Verification items for the finished model (mm, model axes). A direction names the side the tool comes from. Coordinates: 2 decimals unless noted, no trailing zeros. Order: outer loops, then holes, each group sorted by start corner. A loop starts at its lowest first (then second) coordinate and runs counter-clockwise, first axis right, second up. Notation, with made-up numbers: M 37,67 L 76,67 A31 ccw 76,98 Z; hole C 6,4.25 d7. An arc over 180 degrees is marked long. Write item = value, one per line.
```python
from build123d import *

# Parameters (mm, degrees)
F0_R          = 1.5
F1_DEPTH      = 2
F2_W          = 18
F2_H          = 8
F2_W_2        = 14
F2_H_2        = 6
F3_DEPTH      = 14
F4_R          = 0.5
F5_SIZE       = 0.49999
F6_W          = 14
F6_H          = 6
F7_DEPTH      = 2.001
F8_W          = 17
F8_H          = 2
F9_DEPTH      = 3
F9_DEPTH_BACK = 3
F10_W         = 1
F10_H         = 6
F11_DEPTH     = 1
F12_R         = 0.25
F13_DEPTH     = 6.001
F14_W         = 14
F14_H         = 1
F15_DEPTH     = 4


# Not quite as in the source:
# - a fillet or chamfer is up to 0.001 mm smaller than in the source, because OpenCascade refuses the exact size


with BuildPart() as f1:
    # F0 (on Top) → F1 (new body)
    with BuildSketch(Plane.XY):
        with BuildLine():
            Line((20, 4), (0, 4))
            Line((0, 4), (-20, 4))
            ThreePointArc((-20, 4), (-24, 0), (-20, -4))
            Line((-20, -4), (0, -4))
            Line((0, -4), (20, -4))
            ThreePointArc((20, -4), (24, 0), (20, 4))
        make_face()
        with Locations((-20, 0)):
            Circle(F0_R, mode=Mode.SUBTRACT)
        with Locations((20, 0)):
            Circle(F0_R, mode=Mode.SUBTRACT)
    extrude(amount=F1_DEPTH)

    # F2 (on Top) → F3 (join)
    with BuildSketch(Plane.XY):
        Rectangle(F2_W, F2_H)
        Rectangle(F2_W_2, F2_H_2, mode=Mode.SUBTRACT)
    extrude(amount=F3_DEPTH)

    # F4
    f4_edges = [f1.edges().sort_by_distance(p)[0] for p in [
        (9, 0, 2),
        (-9, 0, 2),
        (-9, -4, 8),
        (9, -4, 8),
        (24, 0, 2),
        (14.5, -4, 2),
        (14.5, 4, 2),
        (9, 4, 8),
        (-9, 4, 8),
        (-14.5, -4, 2),
        (-24, 0, 2),
        (-14.5, 4, 2),
    ]]
    fillet(f4_edges, radius=F4_R)

    # F5 (size 0.5 in the source; OpenCascade refuses exactly that, so slightly less here)
    f5_edges = [f1.edges().sort_by_distance(p)[0] for p in [
        (7, 0, 14),
        (0, 3, 14),
        (-7, 0, 14),
        (0, -3, 14),
        (0, -4, 14),
        (0, 4, 14),
        (-8.853553, -3.853553, 14),
        (8.853553, -3.853553, 14),
        (-9, 0, 14),
        (9, 0, 14),
        (-8.853553, 3.853553, 14),
        (8.853553, 3.853553, 14),
    ]]
    chamfer(f5_edges, length=F5_SIZE)

    # F6 (on face) → F7 (cut, through all)
    with BuildSketch(Plane.XY.offset(2)):
        Rectangle(F6_W, F6_H)
    extrude(amount=-F7_DEPTH, mode=Mode.SUBTRACT)

    # F8 (on Front) → F9 (join, two sides)
    with BuildSketch(Plane.XZ) as f9_sk:
        with Locations((0, 5)):
            Rectangle(F8_W, F8_H)
    extrude(amount=-F9_DEPTH)
    extrude(f9_sk.sketch, amount=F9_DEPTH_BACK)

    # F10 (on face) → F11 (join)
    with BuildSketch(Plane.XY.offset(6)):
        with Locations((1.5, 0)):
            Rectangle(F10_W, F10_H)
        with Locations((-4.5, 0)):
            Rectangle(F10_W, F10_H)
    extrude(amount=F11_DEPTH)

    # F12 (on face) → F13 (cut, through all)
    with BuildSketch(Plane.XY.offset(6)):
        with Locations((-2, 1)):
            Circle(F12_R)
        with Locations((-2, -1)):
            Circle(F12_R)
        with Locations((4, 1)):
            Circle(F12_R)
        with Locations((4, -1)):
            Circle(F12_R)
        with Locations((-6, 1)):
            Circle(F12_R)
        with Locations((-6, -1)):
            Circle(F12_R)
    extrude(amount=-F13_DEPTH, mode=Mode.SUBTRACT)

    # F14 (on face) → F15 (join, through all)
    with BuildSketch(Plane(origin=(0, 0, 4), x_dir=(1, 0, 0), z_dir=(0, 0, -1))):
        with Locations((0, -0.056592231)):
            Rectangle(F14_W, F14_H)
    extrude(amount=F15_DEPTH)


solid = f1.part
```
Item 1: Scan lines: L1, parallel to Y at x = -6, z = 4.85; L2, parallel to Y at x = -5.5, z = 2.5; L3, parallel to Y at x = -4, z = 12. Record each from-to range of solid material in increasing order. Write a range as from..to.
Report:
L1 = -4..-1.25, -0.75..0.75, 1.25..4
L2 = -4..-3, -0.44..0.56, 3..4
L3 = -4..-3, 3..4
Item 2: Gauge pin test, flat ends, axial feed: pin 1 (0.5 mm diameter, centred on x = 1.5, y = 0.5, fed in from +Z); pin 2 (2 mm diameter, centred on y = 3, z = 3.5, fed in from -X); pin 3 (2 mm diameter, centred on x = -17, y = 0.5, fed in from +Z); pin 4 (2.5 mm diameter, centred on x = -20, y = 0, fed in from -Z). Record the tip position at first contact, or that the pin passes through.
Report:
pin_1 = 7
pin_2 = -9
pin_3 = 2
pin_4 = through
Item 3: Tool access check on faces 4 (the flat face through (1, 0, 6.5)), 5 (the flat face through (0, -0.443, 2)), 6 (the flat face through (-9, 0, 8)). Record the directions out of +Z, -Z, +X, -X, +Y, -Y that give a thin tool (end or side, any length) a straight path to the whole face; none if there is none.
Report:
face_4 = +Z
face_5 = -Z
face_6 = +Z, -X, +Y, -Y
Item 4: Sectioned sample at A-A, the plane z = 9.25. Enter the section's corners in (x, y), then the cut area to 3 significant figures.
Report:
outline = M -9,-3.5 A0.5 ccw -8.5,-4 L 8.5,-4 A0.5 ccw 9,-3.5 L 9,3.5 A0.5 ccw 8.5,4 L -8.5,4 A0.5 ccw -9,3.5 Z; hole M -7,-3 L 7,-3 L 7,3 L -7,3 Z
area = 59.8 mm^2
Item 5: Sectioned sample at C-C, the plane y = 0. Give the number of separate pieces and of enclosed holes in the cut face, then the cut area to 4 significant figures.
Report:
separate_pieces = 3
enclosed_holes = 0
area = 189.5 mm^2
Item 6: Release check for a two-part mould opening along Y. For faces 1 (the flat face through (0, -4, 5)), 2 (the flat face through (0, 0, 0)), 3 (the cylindrical face through (-21.5, 0.07, 0.99)) record: pulls with the +Y half, pulls with the -Y half, needs draft (parallel to the pull), parting line crosses it, or undercut.
Report:
face_1 = pulls with the -Y half
face_2 = needs draft
face_3 = undercut
Item 7: Sectioned sample at D-D, the plane z = 3.5. Enter the section's corners in (x, y).
Report:
outline = M -9,-3.5 A0.5 ccw -8.5,-4 L 8.5,-4 A0.5 ccw 9,-3.5 L 9,3.5 A0.5 ccw 8.5,4 L -8.5,4 A0.5 ccw -9,3.5 Z; hole M -7,-3 L 7,-3 L 7,-0.44 L -7,-0.44 Z; hole M -7,0.56 L 7,0.56 L 7,3 L -7,3 Z
